from build123d import *

# Parameters (mm, degrees)
F1_DEPTH = 10
F2_W     = 75
F2_H     = 80
F3_DEPTH = 25
F4_W     = 11.9431421733
F4_H     = 45.6254482269
F5_DEPTH = 4
F6_W     = 106.1663627625
F6_H     = 13.160943985
F7_DEPTH = 2.2
F7_TAPER = -3


with BuildPart() as f1:
    # F0 (on Front) → F1 (new body)
    with BuildSketch(Plane.XZ):
        with BuildLine():
            Line((2416.5239715576, -2930.4707694799), (2261.5239715576, -2930.4707694799))
            Line((2261.5239715576, -2930.4707694799), (2261.5239715576, -3180.4707694799))
            Line((2261.5239715576, -3180.4707694799), (2416.5239715576, -3180.4707694799))
            ThreePointArc((2416.5239715576, -3180.4707694799), (2430.6661071813, -3174.6129051036), (2436.5239715576, -3160.4707694799))
            Line((2436.5239715576, -3160.4707694799), (2436.5239715576, -2950.4707694799))
            ThreePointArc((2436.5239715576, -2950.4707694799), (2430.6661071813, -2936.3286338561), (2416.5239715576, -2930.4707694799))
        make_face()
        with BuildLine():
            ThreePointArc((2386.0222752693, -3128.4812615319), (2386.5194053701, -3128.4707703486), (2387.0165433111, -3128.4808831974))
            Line((2387.0165433111, -3128.4808831974), (2396.1245883641, -3128.4774174437))
            ThreePointArc((2396.1245883641, -3128.4774174437), (2396.5194053701, -3128.4707703486), (2396.9142273205, -3128.4771169737))
            ThreePointArc((2396.9142273205, -3128.4771169737), (2405.1461252664, -3132.1246047665), (2408.5239715576, -3140.4707694799))
            ThreePointArc((2408.5239715576, -3140.4707694799), (2405.0091179195, -3148.9561858643), (2396.5235896881, -3152.4707694738))
            Line((2396.5235896881, -3152.4707694738), (2386.6109812809, -3152.4704540302))
            ThreePointArc((2386.6109812809, -3152.4704540302), (2386.5235896881, -3152.4707694738), (2386.4361981155, -3152.4704484682))
            Line((2386.4361981155, -3152.4704484682), (2376.6471792504, -3152.4701369576))
            ThreePointArc((2376.6471792504, -3152.4701369576), (2376.5235896881, -3152.4707694738), (2376.4000001663, -3152.4701290917))
            ThreePointArc((2376.4000001663, -3152.4701290917), (2364.5261998632, -3140.7020147361), (2375.9377122847, -3128.485098866))
            ThreePointArc((2375.9377122847, -3128.485098866), (2376.5194053701, -3128.4707703486), (2377.1011091915, -3128.4846561752))
            Line((2377.1011091915, -3128.4846561752), (2386.0222752693, -3128.4812615319))
        make_face(mode=Mode.SUBTRACT)
        with BuildLine():
            ThreePointArc((2386.1524570887, -3043.476521817), (2386.5310921212, -3043.4707715925), (2386.9097200631, -3043.476971162))
            Line((2386.9097200631, -3043.476971162), (2395.9966068909, -3043.4823631426))
            ThreePointArc((2395.9966068909, -3043.4823631426), (2396.5310921212, -3043.4707715925), (2397.0655632188, -3043.4829974403))
            ThreePointArc((2397.0655632188, -3043.4829974403), (2405.1986214046, -3047.179180366), (2408.5239715576, -3055.4707694799))
            ThreePointArc((2408.5239715576, -3055.4707694799), (2405.0088213897, -3063.9564823743), (2396.5227510032, -3067.4707694178))
            Line((2396.5227510032, -3067.4707694178), (2386.678988276, -3067.4697681805))
            ThreePointArc((2386.678988276, -3067.4697681805), (2386.5227510032, -3067.4707694178), (2386.3665139374, -3067.4697363978))
            Line((2386.3665139374, -3067.4697363978), (2376.7436992517, -3067.4687576337))
            ThreePointArc((2376.7436992517, -3067.4687576337), (2376.5227510032, -3067.4707694178), (2376.3018031686, -3067.4687126872))
            ThreePointArc((2376.3018031686, -3067.4687126872), (2364.5243795036, -3055.3718223336), (2376.4996870262, -3043.4707940523))
            Line((2376.4996870262, -3043.4707940523), (2386.1524570887, -3043.476521817))
        make_face(mode=Mode.SUBTRACT)
        with BuildLine():
            ThreePointArc((2386.4361981157, -2958.4710904915), (2386.5235896881, -2958.4707694859), (2386.6109812808, -2958.4710849295))
            Line((2386.6109812808, -2958.4710849295), (2396.5235896881, -2958.4707694859))
            ThreePointArc((2396.5235896881, -2958.4707694859), (2405.0091179195, -2961.9853530954), (2408.5239715576, -2970.4707694799))
            ThreePointArc((2408.5239715576, -2970.4707694799), (2405.1461252664, -2978.8169341932), (2396.9142273205, -2982.4644219861))
            ThreePointArc((2396.9142273205, -2982.4644219861), (2396.5194053701, -2982.4707686111), (2396.1245883641, -2982.4641215161))
            Line((2396.1245883641, -2982.4641215161), (2387.0165433111, -2982.4606557624))
            ThreePointArc((2387.0165433111, -2982.4606557624), (2386.5194053701, -2982.4707686111), (2386.0222752693, -2982.4602774278))
            Line((2386.0222752693, -2982.4602774278), (2377.1011091916, -2982.4568827845))
            ThreePointArc((2377.1011091916, -2982.4568827845), (2376.5194053701, -2982.4707686111), (2375.9377122847, -2982.4564400938))
            ThreePointArc((2375.9377122847, -2982.4564400938), (2364.5261998632, -2970.2395242236), (2376.4000001663, -2958.471409868))
            ThreePointArc((2376.4000001663, -2958.471409868), (2376.523589688, -2958.4707694859), (2376.6471792503, -2958.4714020022))
            Line((2376.6471792503, -2958.4714020022), (2386.4361981157, -2958.4710904915))
        make_face(mode=Mode.SUBTRACT)
    extrude(amount=F1_DEPTH)

    # F2 (on face) → F3 (cut)
    with BuildSketch(Plane.XZ.offset(10)):
        with Locations((2299.0239715576, -3140.4707694799)):
            Rectangle(F2_W, F2_H)
    extrude(amount=-F3_DEPTH, mode=Mode.SUBTRACT)

    # F4 (on face) → F5 (join)
    with BuildSketch(Plane.XZ.offset(10)):
        with Locations((2387.5132597697, -2971.1128473282)):
            Rectangle(F4_W, F4_H)
    extrude(amount=-F5_DEPTH)

    # F6 (on face) → F7 (cut)
    with BuildSketch(Plane(origin=(0, 0, 0), x_dir=(-1, 0, 0), z_dir=(0, 1, 0))):
        with Locations((-2341.0234451294, -3013.2199525833)):
            Rectangle(F6_W, F6_H)
        with BuildLine():
            ThreePointArc((-2386.4361981157, -2958.4710904915), (-2386.5235896881, -2958.4707694859), (-2386.6109812808, -2958.4710849295))
            Line((-2386.6109812808, -2958.4710849295), (-2396.5235896881, -2958.4707694859))
            ThreePointArc((-2396.5235896881, -2958.4707694859), (-2408.5223126278, -2970.6702978312), (-2396.1245883641, -2982.4641215161))
            Line((-2396.1245883641, -2982.4641215161), (-2387.0165433111, -2982.4606557624))
            ThreePointArc((-2387.0165433111, -2982.4606557624), (-2386.5194053701, -2982.4707686111), (-2386.0222752693, -2982.4602774278))
            Line((-2386.0222752693, -2982.4602774278), (-2377.1011091916, -2982.4568827845))
            ThreePointArc((-2377.1011091916, -2982.4568827845), (-2364.5290948318, -2970.8213865538), (-2376.4000001663, -2958.4714098681))
            ThreePointArc((-2376.4000001663, -2958.471409868), (-2376.523589688, -2958.4707694859), (-2376.6471792503, -2958.4714020022))
            Line((-2376.6471792503, -2958.4714020022), (-2386.4361981157, -2958.4710904915))
        make_face()
    extrude(amount=-F7_DEPTH, taper=F7_TAPER, mode=Mode.SUBTRACT)


solid = f1.part
Can you work these out from the model? Positions are in its coordinate system, mm. A direction names the side the tool comes from. Give positions to 0.01 mm unless a question says otherwise; leave off trailing zeros. Loops run counter-clockwise (first coordinate to the right, second up) from the corner with the lowest first, then second, coordinate; pieces in that order, holes last. Notation, with made-up numbers: M 83,86 L 89,86 A28 ccw 89,107 Z; hole C 87.25,4.5 d1. An arc over 180 degrees is marked long. One line per item, written item: value.
1) Thinking about a two-plate mould opening in X: for faces 1 (the face through (2348, -10, -3026)), 2 (the face through (2430.51, -4.93, -3174.77)), 3 (the face through (2342, -2.2, -3013)), which applies, +X half, -X half, draft (parallel to the pull), parting line (faces both ways), or undercut?
Geometry check:
face 1: draft
face 2: +X half
face 3: undercut
2) On a 3-axis mill with a long thin cutter (end or side, diameter ignored), from which of +Z, -Z, +X, -X, +Y, -Y can I reach the whole of each face in a straight line? I mean faces 4 (the face through (2387, -6, -2970)), 5 (the face through (2336.524, -5, -3141)), 6 (the face through (2436.524, -5, -3057)). Say none if no direction works.
Geometry check:
face 4: +Y
face 5: -Z, -X, +Y, -Y
face 6: +Z, -Z, +X, +Y, -Y
3) Please list where these lines run through material, in increasing order: line 1 (Z direction, x = 2377, y = -1.25); line 2 (Z direction, x = 2390.5, y = -2.5); line 3 (X direction, y = -2, z = -3008).
Geometry check:
line 1: z = -3180.47 to -3152.47, -3128.48 to -3067.47, -3043.47 to -3019.87, -3006.57 to -2982.53, -2958.41 to -2930.47
line 2: z = -3180.47 to -3152.47, -3128.48 to -3067.47, -3043.48 to -2982.46, -2958.47 to -2930.47
line 3: x = 2261.52 to 2287.84, 2394.21 to 2436.52
4) I'm going to push flat-ended pins straight in: pin 1 (5 mm diameter, centred on x = 2294, y = -3, fed in from -Z); pin 2 (8 mm diameter, centred on x = 2370.5, z = -3145.5, fed in from +Y); pin 3 (3.5 mm diameter, centred on x = 2386.5, z = -2968, fed in from +Y). Where does each tip first touch, or does it pass through?
Geometry check:
pin 1: stops at z = -3100.47
pin 2: passes through
pin 3: stops at y = -6
5) Imagine slicing it at C-C on x = 2282. Write out the boundary of the cut face in (y, z).
Geometry check:
outline: M -10,-3100.47 L 0,-3100.47 L 0,-2930.47 L -10,-2930.47 Z
6) Imagine slicing it at D-D on z = -3157.5. Write out the boundary of the cut face in (x, y), and give its area (3 significant figures).
Geometry check:
outline: M 2336.52,-10 L 2436.52,-10 L 2436.52,0 L 2336.52,0 Z
area: 1,000 mm²
7) Imagine slicing it at A-A on y = -3.75. Count the separate pieces of the cut face and the enclosed holes in it, and give its area (3 significant figures).
Geometry check:
separate pieces: 1
enclosed holes: 3
area: 34,800 mm²
